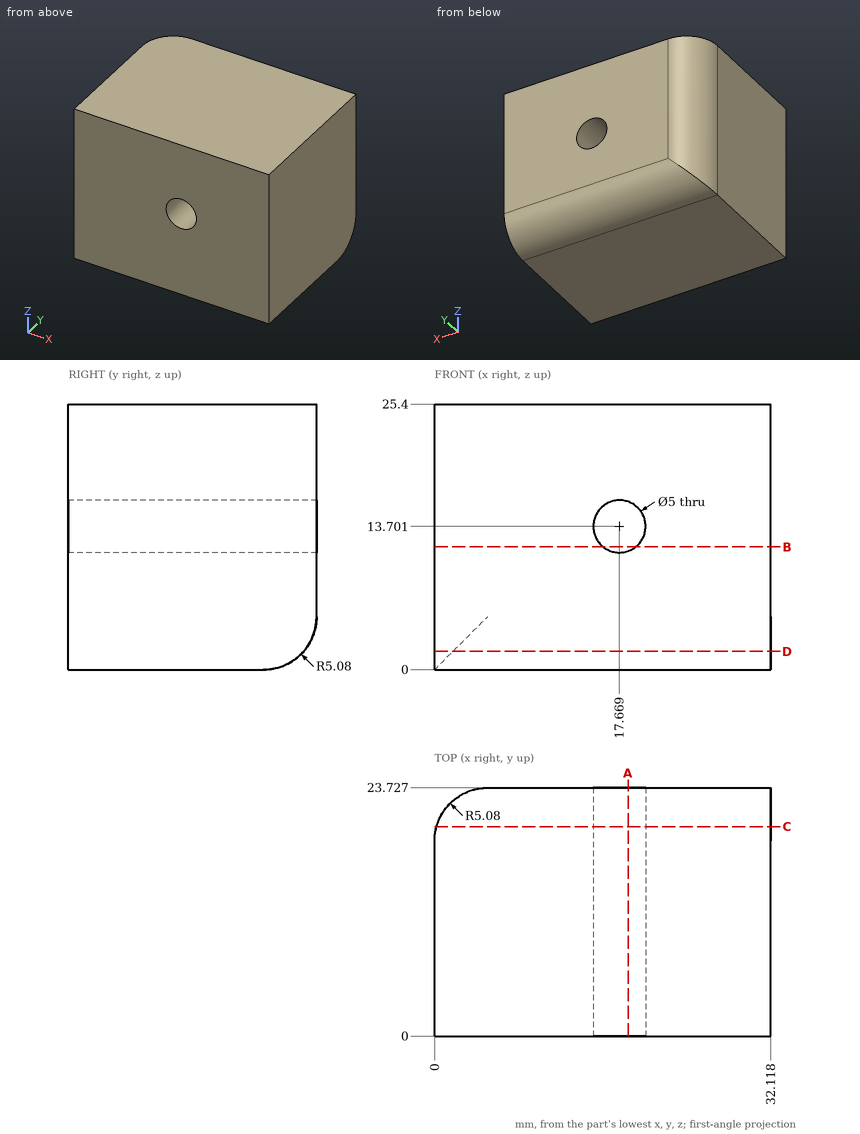
Geometry: see drawing. Coordinates: mm, zero at the bounding-box minimum. Give positions to 0.01 mm unless a question says otherwise; leave off trailing zeros. Order: outer loops, then holes, each group sorted by start corner. A loop starts at its lowest first (then second) coordinate and runs counter-clockwise, first axis right, second up. Notation, with made-up numbers: (69, 69.5) - (82, 69.5) arc R21 cw to (82, 100.5) - close; hole circle Ø8 at (-27, 49.5). An arc over 180 degrees is marked (long way). Use a Markdown table: item, result.
(1) Section query B-B (z = 11.75). Output: boundary loops of the cut face in (x, y).
Computed values:
| item | result |
|---|---|
| outline | (0, 0) - (16.11, 0) - (16.11, 23.73) - (5.08, 23.73) arc R5.08 ccw to (0, 18.65) - close; (19.23, 0) - (32.12, 0) - (32.12, 23.73) - (19.23, 23.73) - close |
(2) Section query D-D (z = 1.75). Output: boundary loops of the cut face in (x, y), then the cut area to 3 significant figures.
Computed values:
| item | result |
|---|---|
| outline | (0, 0) - (32.12, 0) - (32.12, 22.48) - (1.75, 22.48) arc R5.08 ccw to (0, 18.65) - close |
| area | 720 mm2 |
(3) Line query: line 1 (Z direction, x = 16, y = 19) (1 decimal); line 2 (X direction, y = 19.5, z = 13); line 3 (Z direction, x = 18, y = 17.75). Output: solid intervals per line, ascending. Write a range as from..to.
Computed values:
| item | result |
|---|---|
| line 1 | z = 0..11.8, 15.6..25.4 |
| line 2 | x = 0.07..15.27, 20.07..32.12 |
| line 3 | z = 0..11.22, 16.18..25.4 |
(4) Section query A-A (x = 18.5). Output: boundary loops of the cut face in (y, z), then the cut area to 3 significant figures.
Computed values:
| item | result |
|---|---|
| outline | (0, 0) - (18.65, 0) arc R5.08 ccw to (23.73, 5.08) - (23.73, 11.34) - (0, 11.34) - close; (0, 16.06) - (23.73, 16.06) - (23.73, 25.4) - (0, 25.4) - close |
| area | 485 mm2 |
(5) Section query C-C (y = 20). Output: boundary loops of the cut face in (x, z), then the cut area to 3 significant figures.
Computed values:
| item | result |
|---|---|
| outline | (0.18, 0.18) - (32.12, 0.18) - (32.12, 25.4) - (0.18, 25.4) - close; hole circle Ø5 at (17.67, 13.7) |
| area | 786 mm2 |
